Check sheet for the modelled part. Datum: model origin and axes. Units: mm. Face numbers are marked on the shaded views. A direction names the side the tool comes from. Round coordinates to 2 decimals unless told otherwise and drop trailing zeros. Write each loop counter-clockwise with the first axis right and the second up, starting at its lowest first coordinate (ties: lowest second). Pieces come first, ordered by that corner, then holes. Notation, with made-up numbers: (-23, 68) -> (27, 68) arc R9 ccw to (27, 81) -> close; hole circle Ø4 at (88, -17.5). An arc over 180 degrees is marked (long way). Put each result on its own line as item: value. Start each with the question number.
from build123d import *
from build123d.topology import SkipClean

# Parameters (mm, degrees)
BOSS_EXTRUDE1_DEPTH = 15
BOSS_EXTRUDE2_DEPTH = 21
SKETCH4_W           = 10.2
SKETCH4_H           = 2.9999999999999964
CUT_EXTRUDE1_DEPTH  = 62.298960023804646
SKETCH9_R           = 10.5
CUT_EXTRUDE6_DEPTH  = 62.298960023804646
SKETCH5_W           = 10.2
SKETCH5_H           = 3
CUT_EXTRUDE2_DEPTH  = 73.85087508053697
BOSS_EXTRUDE4_REACH = 51.095
SKETCH10_W          = 5
SKETCH10_H          = 5.5837661042678555
CUT_EXTRUDE7_DEPTH  = 5
SKETCH6_R           = 2.7
CUT_EXTRUDE3_DEPTH  = 14.4
CUT_EXTRUDE4_DEPTH  = 50.09503539055656
SKETCH8_W           = 5
SKETCH8_H           = 16.75
CUT_EXTRUDE5_DEPTH  = 35
SKETCH12_R          = 2.7
CUT_EXTRUDE8_DEPTH  = 5
SKETCH13_R          = 2.7
CUT_EXTRUDE9_DEPTH  = 75.801403730144
FILLET1_R           = 5
FILLET2_R           = 1


with BuildPart() as part:
    # Sketch2 → Boss-Extrude1 (new body)
    with BuildSketch(Plane(origin=(0, 0, 0), x_dir=(0, 0, -1), z_dir=(1, 0, 0))):
        Polygon((0, 24.75), (-6.7, 24.75), (-22.4, 15.685600773722843), (-22.399999999999995, -2.156584454693771), (-43, -14.050000000000002), (-43, -24.75), (0, -24.75), align=None)
    extrude(amount=BOSS_EXTRUDE1_DEPTH)

    # Sketch3 → Boss-Extrude2 (add)
    with BuildSketch(Plane(origin=(15, 0, 0), x_dir=(0, 0, -1), z_dir=(1, 0, 0))):
        Polygon((-22.4, 15.685600773722843), (-22.4, -5.192264973080983), (-14.5, -9.753332099679069), (0, -9.753332099679069), (0, 20.246667900320933), (-14.5, 20.246667900320933), align=None)
    extrude(amount=BOSS_EXTRUDE2_DEPTH)

    # Sketch4 → Cut-Extrude1 (cut, through all)
    with BuildSketch(Plane.XY.offset(43)):
        with Locations((5.1, -23.25)):
            Rectangle(SKETCH4_W, SKETCH4_H)
    extrude(amount=-CUT_EXTRUDE1_DEPTH, mode=Mode.SUBTRACT)

    # Sketch9 → Cut-Extrude6 (cut, through all)
    with BuildSketch(Plane(origin=(36.00000000000001, 0, 0), x_dir=(0, 0, -1), z_dir=(1, 0, 0))):
        with Locations((-15, 5.24666790032093)):
            Circle(SKETCH9_R)
    extrude(amount=-CUT_EXTRUDE6_DEPTH, mode=Mode.SUBTRACT)

    # Sketch5 → Cut-Extrude2 (cut, through all)
    with BuildSketch(Plane.XZ.offset(21.750000000000004)):
        with Locations((5.1, 1.5)):
            Rectangle(SKETCH5_W, SKETCH5_H)
    extrude(amount=-CUT_EXTRUDE2_DEPTH, mode=Mode.SUBTRACT)

    # Boss-Extrude4: up to this face of the body (flat: up to its plane)
    boss_extrude4_end = Plane(part.part.faces().sort_by_distance((5.1, 1.5, 3))[0])
    # Sketch10 → Boss-Extrude4 (add, up to the picked face)
    with BuildSketch(Plane.XY.offset(22.399999999999995), mode=Mode.PRIVATE) as boss_extrude4_sk1:
        with Locations((2.5, 15.48771197904034)):
            Rectangle(SKETCH10_W, SKETCH10_H)
    boss_extrude4_tool1 = split(extrude(boss_extrude4_sk1.sketch, amount=-BOSS_EXTRUDE4_REACH, mode=Mode.PRIVATE), bisect_by=boss_extrude4_end, keep=Keep.BOTH, mode=Mode.PRIVATE)
    add(boss_extrude4_tool1.solids().sort_by(Axis((2.5, 15.487712, 22.4), (0, 0, -1)))[0])

    # Sketch11 → Cut-Extrude7 (cut)
    with BuildSketch(Plane(origin=(5, 0, 0), x_dir=(0, 0, -1), z_dir=(1, 0, 0))):
        Polygon((-22.399999999999995, 15.685600773722847), (-17.907070151552254, 18.279595031174264), (-22.399999999999995, 18.279595031174264), align=None)
    extrude(amount=-CUT_EXTRUDE7_DEPTH, mode=Mode.SUBTRACT)

    # Sketch6 → Cut-Extrude3 (cut)
    with BuildSketch(Plane.XY.offset(22.399999999999995)):
        with BuildLine():
            Line((5, 19.250000000000004), (5.000000000000001, 24.750000000000004))
            Line((5.000000000000001, 24.750000000000004), (-5, 24.750000000000004))
            Line((-5, 24.750000000000004), (-5, 19.250000000000004))
            ThreePointArc((-5, 19.250000000000004), (-9.2e-16, 14.250000000000004), (5, 19.250000000000004))
        make_face()
        with Locations((0, 19.250000000000004)):
            Circle(SKETCH6_R, mode=Mode.SUBTRACT)
    extrude(amount=-CUT_EXTRUDE3_DEPTH, mode=Mode.SUBTRACT)

    # Sketch7 → Cut-Extrude4 (cut, through all)
    with BuildSketch(Plane.XY.offset(22.399999999999995)):
        with BuildLine():
            Line((0, 21.950000000000006), (0, 16.549999999999997))
            ThreePointArc((0, 16.549999999999997), (2.7000000000000064, 19.250000000000004), (0, 21.950000000000006))
        make_face()
    extrude(amount=-CUT_EXTRUDE4_DEPTH, mode=Mode.SUBTRACT)

    # Sketch8 → Cut-Extrude5 (cut)
    with BuildSketch(Plane.XY.offset(43)):
        with Locations((2.5, -8.375)):
            Rectangle(SKETCH8_W, SKETCH8_H)
    extrude(amount=-CUT_EXTRUDE5_DEPTH, mode=Mode.SUBTRACT)

    # Sketch12 → Cut-Extrude8 (cut)
    with BuildSketch(Plane.XY.offset(8)):
        with Locations((0, -11.750000000000002)):
            Circle(SKETCH12_R)
    extrude(amount=-CUT_EXTRUDE8_DEPTH, mode=Mode.SUBTRACT)

    # Sketch13 → Cut-Extrude9 (cut, through all)
    with BuildSketch(Plane(origin=(0, 24.75, 0), x_dir=(1, 0, 0), z_dir=(0, 1, 0))):
        with Locations((0, -15.5)):
            Circle(SKETCH13_R)
        with BuildLine():
            Line((2.7, -35.5), (2.7000000000000006, -43))
            Line((2.7000000000000006, -43), (-2.7000000000000006, -43))
            Line((-2.7000000000000006, -43), (-2.7, -35.5))
            ThreePointArc((-2.7, -35.5), (1.7e-16, -32.8), (2.7, -35.5))
        make_face()
    extrude(amount=-CUT_EXTRUDE9_DEPTH, mode=Mode.SUBTRACT)

    # Fillet1
    fillet1_edges = [part.edges().sort_by_distance(p)[0] for p in [
        (25.5, 20.246667900320933, 14.5),
        (25.5, -9.753332099679069, 14.5),
        (7.5, 24.75, 6.7),
    ]]
    fillet(fillet1_edges, radius=FILLET1_R)

    # Fillet2
    fillet2_edges = [part.edges().sort_by_distance(p)[0] for p in [
        (15, 24.75, 2.6801270189221915),
        (15, 24.57962913144534, 6.654349263356993),
        (36, 20.246667900320933, 6.580127018922168),
        (36, 20.07629703176627, 14.454349263356942),
        (36, -9.753332099679069, 6.5801270189221865),
        (36, -9.582961231124408, 14.454349263356988),
        (15, 21.828460969082656, 11.760254037844366),
        (36, 17.63119784648299, 19.030127018922176),
        (36, -7.137862045841118, 19.030127018922194),
        (10.2, -24.75, 21.5),
        (15, -24.75, 21.5),
        (15, -8.11170848370516, 32.71457738362205),
    ]]
    fillet(fillet2_edges, radius=FILLET2_R)

    # Mirror1: part across plane


with BuildPart() as part_1:
    with SkipClean():  # the faces are left unmerged after this step: merging them gives an invalid solid
        add(part.part)
        add(part.part.mirror(Plane(origin=(0, 0, 0), x_dir=(0, 0, 1), z_dir=(1, 0, 0))))


solid = part_1.part
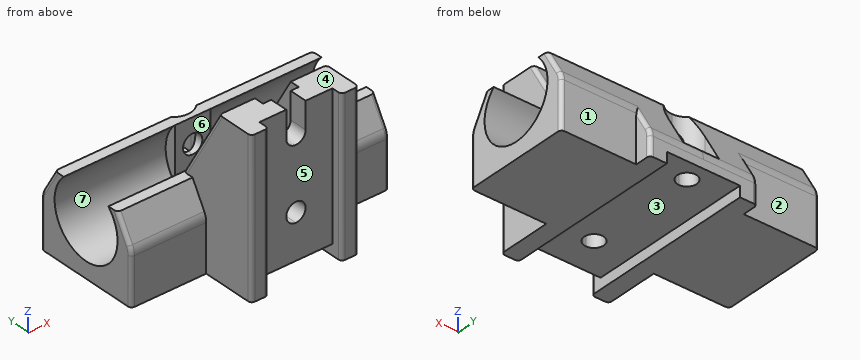
1. Access from +Z, -Z, +X, -X, +Y, -Y to the whole of each face (thin tool, end or side, straight path). Record for the marked faces 1, 2 and 3.
2. Gauge pin test, flat ends, axial feed: P1, Ø12, axis at y = -7.5, z = 29.5, coming from the +X side; P2, Ø6, axis at x = 5, z = 27, coming from the -Y side; P3, Ø10, axis at x = -12, z = 37, coming from the +Y side. Record the tip position at first contact, or that the pin passes through.
3. Material ranges on L1, parallel to X at y = -16.5, z = 17.5; L2, parallel to X at y = -18, z = 38; L3, parallel to Z at x = -6.5, y = -3, recorded low to high. Write a range as [from, to].
4. Section check C-C, the plane x = -29.5. Enter the section's corners in (y, z), then the cut area to 3 significant figures.
5. Section check A-A, the plane x = 12. Enter the section's corners in (y, z), then the cut area to 3 significant figures.
6. Draft check along Y on the marked faces 4, 5, 6 and 7. Enter one of: released by +Y, released by -Y, zero draft, split by the parting line, or undercut.
7. Section check B-B, the plane z = 14. Give the number of separate pieces and of enclosed holes in the cut face, then the cut area to 3 significant figures.
Reply:
1. face 1: +Z, -Z, +X, +Y
1. face 2: +Z, -Z, -X, +Y
1. face 3: -Z, +Y, -Y
2. P1: stops at x = 15
2. P2: stops at y = -21.75
2. P3: stops at y = -7.7
3. L1: x = [-15, -5], [5, 15]
3. L2: x = [-15, -2.7], [2.7, 15]
3. L3: z = [3, 8.5], [21.5, 23.86]
4. outline: (-9.75, 0) -> (20.25, 0) -> (20.25, 13.16) arc R5 ccw to (19.58, 15.66) -> (15.69, 22.4) -> (12.7, 22.4) arc R10.5 cw (long way) to (-2.2, 22.4) -> (-5.19, 22.4) -> (-9.08, 15.66) arc R5 ccw to (-9.75, 13.16) -> close
4. area: 321 mm2
5. outline: (-24.75, 0) -> (24.75, 0) -> (24.75, 5.36) arc R5 ccw to (24.08, 7.86) -> (15.69, 22.4) -> (12.7, 22.4) arc R10.5 cw (long way) to (-2.17, 22.43) -> (-14.05, 43) -> (-24.75, 43) -> close
5. area: 1,070 mm2
6. face 4: zero draft
6. face 5: released by -Y
6. face 6: undercut
6. face 7: undercut
7. separate pieces: 4
7. enclosed holes: 0
7. area: 876 mm2
